Could you check a few things on this model? Use its own coordinates, in mm. Round coordinates to 2 decimals unless told otherwise and drop trailing zeros. Loops run counter-clockwise (first coordinate to the right, second up) from the corner with the lowest first, then second, coordinate; pieces in that order, holes last. Notation, with made-up numbers: (56, 49.25) - (66, 49.25) arc R20 ccw to (66, 55.25) - close; hole circle Ø7 at (-12.75, 70). An arc over 180 degrees is marked (long way). Answer as CSV lines item,"result". Start each with the question number.
1) Suppose I cut it at C-C, the plane y = -0.25. Write out the boundary of the cut face in (x, z).
2) Suppose I cut it at B-B, the plane x = 0. Write out the boundary of the cut face in (y, z) (3 decimals), then the cut area to 3 significant figures.
3) Suppose I cut it at A-A, the plane x = 19.85. Write out the boundary of the cut face in (y, z), then the cut area to 3 significant figures.
4) Please list where these lines run through material, in increasing order: line 1 along Y through (x, z) = (19.85, 3.6); line 2 along Y through (x, z) = (-15.5, 3.7) (3 decimals); line 3 along X through (y, z) = (50.5, 2.1).
5) Suppose I cut it at D-D, the plane y = 23. Write out the boundary of the cut face in (x, z).
6) I'm going to push a flat-ended pin straight in: pin 1 Ø9 at (x, y) = (19.85, -0.25) entering from +Z. Where does the tip first touch, or does it pass through?
```python
from build123d import *

# Parameters (mm, degrees)
SKETCH1_W           = 65.5
SKETCH1_H           = 110
BOSS_EXTRUDE1_DEPTH = 5
SKETCH2_R           = 12.5
CUT_EXTRUDE1_DEPTH  = 65.207184177
SKETCH3_R           = 1.65
CUT_EXTRUDE2_DEPTH  = 65.207184177
SKETCH4_R           = 2.75
CUT_EXTRUDE3_DEPTH  = 65.207184177


with BuildPart() as part:
    # Sketch1 → Boss-Extrude1 (new body)
    with BuildSketch(Plane.XY):
        Rectangle(SKETCH1_W, SKETCH1_H)
    extrude(amount=BOSS_EXTRUDE1_DEPTH)

    # Sketch2 → Cut-Extrude1 (cut, through all)
    with BuildSketch(Plane(origin=(0, 0, 0), x_dir=(-1, 0, 0), z_dir=(0, 0, -1))):
        with Locations((0, 34.025)):
            Circle(SKETCH2_R)
    extrude(amount=-CUT_EXTRUDE1_DEPTH, mode=Mode.SUBTRACT)

    # Sketch3 → Cut-Extrude2 (cut, through all)
    with BuildSketch(Plane(origin=(0, 0, 0), x_dir=(-1, 0, 0), z_dir=(0, 0, -1))):
        with Locations((-15.5, 49.525)):
            Circle(SKETCH3_R)
        with Locations((-15.5, 18.525)):
            Circle(SKETCH3_R)
        with Locations((15.5, 18.525)):
            Circle(SKETCH3_R)
        with Locations((15.5, 49.525)):
            Circle(SKETCH3_R)
    extrude(amount=-CUT_EXTRUDE2_DEPTH, mode=Mode.SUBTRACT)

    # Sketch4 → Cut-Extrude3 (cut, through all)
    with BuildSketch(Plane(origin=(0, 0, 0), x_dir=(-1, 0, 0), z_dir=(0, 0, -1))):
        with Locations((-19.85, -0.25)):
            Circle(SKETCH4_R)
        with Locations((19.85, -0.25)):
            Circle(SKETCH4_R)
        with Locations((19.85, -42.25)):
            Circle(SKETCH4_R)
        with Locations((-19.85, -42.25)):
            Circle(SKETCH4_R)
    extrude(amount=-CUT_EXTRUDE3_DEPTH, mode=Mode.SUBTRACT)


solid = part.part
```
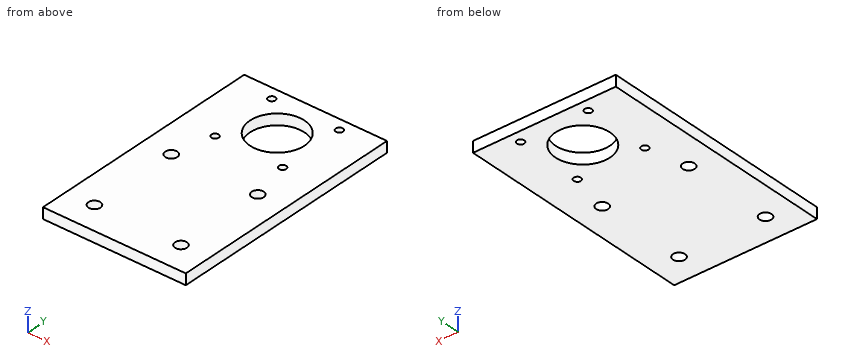
Filled sheet:
1,outline,"(-32.75, 0) - (-22.6, 0) - (-22.6, 5) - (-32.75, 5) - close; (-17.1, 0) - (17.1, 0) - (17.1, 5) - (-17.1, 5) - close; (22.6, 0) - (32.75, 0) - (32.75, 5) - (22.6, 5) - close"
2,outline,"(-55, 0) - (21.525, 0) - (21.525, 5) - (-55, 5) - close; (46.525, 0) - (55, 0) - (55, 5) - (46.525, 5) - close"
2,area,"425 mm²"
3,outline,"(-55, 0) - (-45, 0) - (-45, 5) - (-55, 5) - close; (-39.5, 0) - (-3, 0) - (-3, 5) - (-39.5, 5) - close; (2.5, 0) - (55, 0) - (55, 5) - (2.5, 5) - close"
3,area,"495 mm²"
4,line 1,"-55 to -45, -39.5 to -3, 2.5 to 55"
4,line 2,"-55 to 16.875, 20.175 to 47.875, 51.175 to 55"
4,line 3,"-32.75 to -16.83, -14.17 to 14.17, 16.83 to 32.75"
5,outline,"(-32.75, 0) - (-5.89, 0) - (-5.89, 5) - (-32.75, 5) - close; (5.89, 0) - (32.75, 0) - (32.75, 5) - (5.89, 5) - close"
6,pin 1,"z = 5"
